```python
from build123d import *

# Parameters (mm, degrees)
PAD017_DEPTH           = 5
PAD020_DEPTH           = 6.25
SKETCH038_W            = 10
SKETCH038_H            = 1.65
PAD021_DEPTH           = 5
SKETCH085_W            = 10
SKETCH085_H            = 1.65
PAD054_DEPTH           = 7.5
SKETCH083_W            = 7.1
SKETCH083_H            = 1.65
PAD055_DEPTH           = 7.5
SKETCH082_W            = 10
SKETCH082_H            = 1.65
PAD056_DEPTH           = 4.6
SKETCH084_W            = 10
SKETCH084_H            = 1.65
PAD057_DEPTH           = 7.5
LINEARPATTERN019_COUNT = 2
LINEARPATTERN019_PITCH = 3.3
CHAMFER009_SIZE        = 1


with BuildPart() as obj1:
    # Sketch034 → Pad017 (new body)
    with BuildSketch(Plane.XY):
        with BuildLine():
            Line((-1.35, -1.8), (-1.35, 6))
            ThreePointArc((0, 7.35), (-0.954594, 6.954594), (-1.35, 6))
            Line((0, 9), (0, 7.35))
            Line((-2.6, 9), (0, 9))
            Line((-2.6, -1.8), (-2.6, 9))
            Line((-3.85, -1.8), (-2.6, -1.8))
            ThreePointArc((-3.85, -1.8), (-3.439949, -2.789949), (-2.45, -3.2))
            Line((-1.35, -3.2), (-2.45, -3.2))
            Line((-1.35, -1.8), (-1.35, -3.2))
        make_face()
    extrude(amount=PAD017_DEPTH)

    # Sketch037 → Pad020 (join)
    with BuildSketch(Plane.XY):
        Polygon((-1.35, 0.2), (-1.35, 1.6), (-2.6, 1.6), (-3.85, 1.6), (-3, 0.2), (-2.6, 0.2), align=None)
    extrude(amount=PAD020_DEPTH)


with BuildPart() as body030:
    # Mirror002: instance of _obj1
    add(obj1.part.mirror(Plane(origin=(5, 0, 0), x_dir=(0, 1, 0), z_dir=(-1, 0, 0))))

    # Fusion002: union _obj1
    add(obj1.part)


with BuildPart() as body030_1:
    # Clone003 placement: moved
    add(body030.part.moved(Location((-5, 0, 0))))

    # Sketch038 → Pad021 (new body)
    with BuildSketch(Plane.XY):
        with Locations((0, 8.175)):
            Rectangle(SKETCH038_W, SKETCH038_H)
    extrude(amount=PAD021_DEPTH)

    # Sketch085 → Pad054 (new body)
    with BuildSketch(Plane.XY):
        with Locations((2.6, 8.175)):
            Rectangle(SKETCH085_W, SKETCH085_H)
    extrude(amount=PAD054_DEPTH)

    # Sketch083 → Pad055 (join)
    with BuildSketch(Plane.XY):
        with Locations((4.05, 9.825)):
            Rectangle(SKETCH083_W, SKETCH083_H)
    pad055 = extrude(amount=PAD055_DEPTH)

    # Sketch082 → Pad056 (join)
    with BuildSketch(Plane.XY):
        with Locations((2.6, 9.825)):
            Rectangle(SKETCH082_W, SKETCH082_H)
    pad056 = extrude(amount=PAD056_DEPTH)

    # Sketch084 → Pad057 (join)
    with BuildSketch(Plane.XY):
        with Locations((2.6, 11.475)):
            Rectangle(SKETCH084_W, SKETCH084_H)
    pad057 = extrude(amount=PAD057_DEPTH)

    # LinearPattern019: Pad057, Pad056, Pad055 ×2
    with Locations(*[(0, i * LINEARPATTERN019_PITCH, 0) for i in range(1, LINEARPATTERN019_COUNT)]):
        add(pad057)
        add(pad056)
        add(pad055)

    # Chamfer009
    chamfer009_edges = [body030_1.edges().sort_by_distance(p)[0] for p in [
        (-2.4, 8.175, 7.5),
        (-2.4, 11.475, 7.5),
        (-2.4, 14.775, 7.5),
    ]]
    chamfer(chamfer009_edges, length=CHAMFER009_SIZE)


with BuildPart() as body030_2:
    # Body030 placement: moved
    add(body030_1.part.moved(Location((-5, 0, 0))))


solid = body030_2.part
```
For this review, take the finished solid that the model builds, in its own axes (mm). A direction names the side the tool comes from. Coordinates: 2 decimals unless noted, no trailing zeros. Write each loop counter-clockwise with the first axis right and the second up, starting at its lowest first coordinate (ties: lowest second). Pieces come first, ordered by that corner, then holes.
(1) Wall thickness on probe 1 along X at (y, z) = (4.75, 2.75); probe 2 along Y at (x, z) = (-5.75, 0.5); probe 3 along X at (y, z) = (12.5, 4.5): over which ranges is each line inside the solid? List them lowest first.
(2) Add section A-A on y = 3.25. Give the boundary of the cut face in (x, z), then the cut area to 3 significant figures.
(3) For pin 1 Ø2.5 at (x, z) = (-5.5, 6) entering from -Y; pin 2 Ø0.8 at (x, y) = (1, 5) entering from +Z; pin 3 Ø2 at (y, z) = (4.5, 2.5) entering from -X, all flat-tipped, find the tip position at first contact; note any pin that passes through.
(4) The part is to be moulded in two halves that separate along Y. For faces 5 (the face through (-6.9, 8.2, 7)), 6 (the face through (-6, 13.95, 6)), 7 (the face through (-12, -3.2, 2)), say which applies: +Y half, -Y half, draft (parallel to the pull), parting line (faces both ways), or undercut.
(5) Tool access review of faces 1 (the face through (2, -2, 5)), 2 (the face through (2.6, -1, 2)), 3 (the face through (-13, -1.8, 2)), 4 (the face through (2, 5, 5)): name each direction out of +Z, -Z, +X, -X, +Y, -Y from which nothing blocks a thin tool from reaching the whole face with its end or side.
(6) Add section C-C on z = 2.5. Give the boundary of the cut face in (x, y).
(7) Add section B-B on z = 5.5. Give the boundary of the cut face in (x, y), then the cut area to 3 significant figures.
(8) Add section D-D on y = 11. Give the boundary of the cut face in (x, z).
Answer sheet:
1. probe 1: x = -12.6 to -11.35, 1.35 to 2.6
1. probe 2: y = 7.35 to 15.6
1. probe 3: x = -7.4 to 2.6
2. outline: (-12.6, 0) - (-11.35, 0) - (-11.35, 5) - (-12.6, 5) - close; (1.35, 0) - (2.6, 0) - (2.6, 5) - (1.35, 5) - close
2. area: 12.5 mm2
3. pin 1: stops at y = 7.35
3. pin 2: stops at z = 5
3. pin 3: stops at x = -12.6
4. face 5: draft
4. face 6: undercut
4. face 7: -Y half
5. face 1: +Z, +X, -X, -Y
5. face 2: +Z, -Z, +X
5. face 3: +Z, -Z, -X
5. face 4: +Z, +X, -X
6. outline: (-13.85, -1.8) arc R1.4 ccw to (-12.45, -3.2) - (-11.35, -3.2) - (-11.35, 6) arc R1.35 cw to (-10, 7.35) - (0, 7.35) arc R1.35 cw to (1.35, 6) - (1.35, -3.2) - (2.45, -3.2) arc R1.4 ccw to (3.85, -1.8) - (2.6, -1.8) - (2.6, 0.2) - (3, 0.2) - (3.85, 1.6) - (2.6, 1.6) - (2.6, 15.6) - (-7.4, 15.6) - (-7.4, 9) - (-12.6, 9) - (-12.6, 1.6) - (-13.85, 1.6) - (-13, 0.2) - (-12.6, 0.2) - (-12.6, -1.8) - close
7. outline: (-13.85, 1.6) - (-13, 0.2) - (-11.35, 0.2) - (-11.35, 1.6) - close; (-7.4, 7.35) - (2.6, 7.35) - (2.6, 15.6) - (-7.4, 15.6) - (-7.4, 13.95) - (-4.5, 13.95) - (-4.5, 12.3) - (-7.4, 12.3) - (-7.4, 10.65) - (-4.5, 10.65) - (-4.5, 9) - (-7.4, 9) - close; (1.35, 0.2) - (3, 0.2) - (3.85, 1.6) - (1.35, 1.6) - close
7. area: 78.7 mm2
8. outline: (-7.4, 0) - (2.6, 0) - (2.6, 7.5) - (-6.4, 7.5) - (-7.4, 6.5) - close
